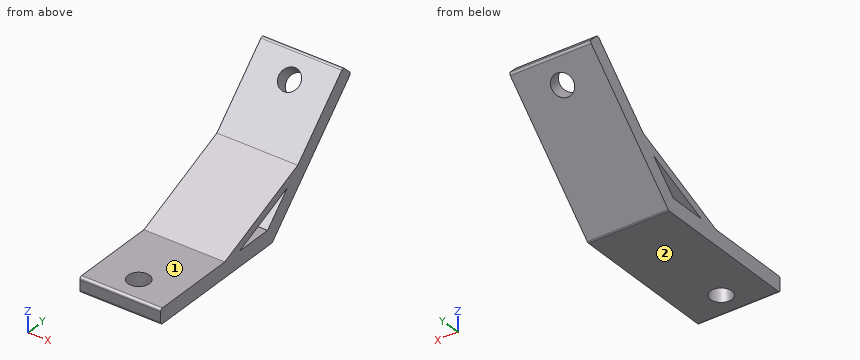
from build123d import *

# Parameters (mm, degrees)
PAD_DEPTH       = 16
SKETCH001_R     = 4.25
POCKET_DEPTH    = 6
SKETCH002_R     = 4.25
POCKET001_DEPTH = 6
FILLET_R        = 1


with BuildPart() as part:
    # Sketch → Pad (new body, symmetric)
    with BuildSketch(Plane.YZ):
        Polygon((-60, 0), (0, 0), (42.4264068712, 42.4264068712), (38.1837661841, 46.6690475583), (13.7781745931, 22.2634559673), (-25.4852813742, 6), (-60, 6), align=None)
        Polygon((8.1213203436, 16.6066017178), (-17.4852813742, 6), (-2.4852813742, 6), align=None, mode=Mode.SUBTRACT)
    extrude(amount=PAD_DEPTH, both=True)

    # Sketch001 (on Face6 of Pad) → Pocket (cut)
    with BuildSketch(Plane(origin=(0, 0, 6), x_dir=(0, -1, 0), z_dir=(0, 0, 1))):
        with Locations((50, 0)):
            Circle(SKETCH001_R)
    extrude(amount=-POCKET_DEPTH, mode=Mode.SUBTRACT)

    # Sketch002 (on Face9 of Pocket) → Pocket001 (cut)
    with BuildSketch(Plane(origin=(0, -4.2426406871, 4.2426406871), x_dir=(0, -0.7071067812, -0.7071067812), z_dir=(0, -0.7071067812, 0.7071067812))):
        with Locations((-50, 0)):
            Circle(SKETCH002_R)
    extrude(amount=-POCKET001_DEPTH, mode=Mode.SUBTRACT)

    # Fillet
    fillet_edges = [part.edges().sort_by_distance(p)[0] for p in [
        (0, 0, 0),
        (0, -60, 0),
        (0, -60, 6),
        (0, 38.183766, 46.669048),
        (0, 42.426407, 42.426407),
    ]]
    fillet(fillet_edges, radius=FILLET_R)


solid = part.part
Geometry check sheet. Reference: the model listing, model coordinates, mm. Face numbers are marked on the shaded views. A direction names the side the tool comes from. Give positions to 0.01 mm unless a question says otherwise; leave off trailing zeros. Write each loop counter-clockwise with the first axis right and the second up, starting at its lowest first coordinate (ties: lowest second). Pieces come first, ordered by that corner, then holes. Notation, with made-up numbers: M 84.5,19 L 99.5,19 A13 cw 99.5,33 Z; hole C 64.25,77 d6. An arc over 180 degrees is marked long. One line per question, with ' | ' between items.
1. Set-up check for the marked faces 1 and 2: record each of +Z, -Z, +X, -X, +Y, -Y from which the full face is reachable in a straight line by a thin tool's end or side.
Ans:
face 1: +Z, +X, -X, -Y | face 2: -Z, +X, -X, +Y, -Y
2. Cross-section at A-A (y = -50). Enter the section's corners in (x, z).
Ans:
outline: M -16,0 L -4.25,0 L -4.25,6 L -16,6 Z; M 4.25,0 L 16,0 L 16,6 L 4.25,6 Z
3. Cross-section at B-B (x = -1.5). Enter the section's corners in (y, z), plus the area to 3 significant figures.
Ans:
outline: M -60,1 A1 ccw -59,0 L -53.98,0 L -53.98,6 L -59,6 A1 ccw -60,5 Z; M -46.02,0 L -0.41,0 A1 ccw 0.29,0.29 L 32.54,32.54 L 28.3,36.79 L 13.78,22.26 L -25.49,6 L -46.02,6 Z; M 33.92,42.41 L 38.17,38.17 L 41.72,41.72 A1 ccw 41.72,43.13 L 38.89,45.96 A1 ccw 37.48,45.96 Z; hole M -17.49,6 L -2.49,6 L 8.12,16.61 Z | area: 716 mm2
4. Cross-section at D-D (x = 13). Enter the section's corners in (y, z), plus the area to 3 significant figures.
Ans:
outline: M -60,1 A1 ccw -59,0 L -0.41,0 A1 ccw 0.29,0.29 L 41.72,41.72 A1 ccw 41.72,43.13 L 38.89,45.96 A1 ccw 37.48,45.96 L 13.78,22.26 L -25.49,6 L -59,6 A1 ccw -60,5 Z; hole M -17.49,6 L -2.49,6 L 8.12,16.61 Z | area: 812 mm2
5. Gauge pin test, flat ends, axial feed: pin 1 (12 mm diameter, centred on x = 9, y = 15.5, fed in from +Z); pin 2 (8 mm diameter, centred on x = 8, z = 35, fed in from -Y); pin 3 (16.5 mm diameter, centred on x = 5.5, y = -8.5, fed in from +Z). Record the tip position at first contact, or that the pin passes through.
Ans:
pin 1: z = 29.99 | pin 2: y = 22.51 | pin 3: z = 16.45
6. Scan lines: line 1 along X through (y, z) = (-50, 3.15); line 2 along Z through (x, y) = (7, -38.5); line 3 along Z through (x, y) = (4, -10.5). Record each from-to range of solid material in increasing order. Write a range as from..to.
Ans:
line 1: -16..-4.25, 4.25..16 | line 2: 0..6 | line 3: 0..6, 8.89..12.21
7. Cross-section at C-C (z = 4). Enter the section's corners in (x, y).
Ans:
outline: M -16,-60 L 16,-60 L 16,4 L -16,4 Z; hole C 0,-50 d8.5
